Verification items for the finished model (mm, model axes). Face numbers are marked on the shaded views. Round coordinates to 2 decimals unless told otherwise and drop trailing zeros. Order: outer loops, then holes, each group sorted by start corner. A loop starts at its lowest first (then second) coordinate and runs counter-clockwise, first axis right, second up. Notation, with made-up numbers: M 62,6.25 L 66,6.25 A24 cw 66,44.25 Z; hole C 72.25,-4 d8. An arc over 180 degrees is marked long. Answer as a JSON object with one key per item and string values. Group by question number.
```python
from build123d import *

# Parameters (mm, degrees)
F1_DEPTH  = 7.1
F2_T      = -2.5
F4_DEPTH  = 25
F5_W      = 12.5
F5_H      = 1.25
F6_DEPTH  = 2.5
F7_W      = 23.5
F7_H      = 1.25
F8_DEPTH  = 2.5
F9_W      = 1.5
F9_H      = 7.25
F9_R      = 2.5
F10_DEPTH = 4.4


with BuildPart() as f1:
    # F0 (on Front) → F1 (new body)
    with BuildSketch(Plane.XZ):
        with BuildLine():
            Line((68.55, 39.5), (-68.55, 39.5))
            ThreePointArc((-68.55, 39.5), (-72.72193, 37.77193), (-74.45, 33.6))
            Line((-74.45, 33.6), (-74.45, -33.6))
            ThreePointArc((-74.45, -33.6), (-72.72193, -37.77193), (-68.55, -39.5))
            Line((-68.55, -39.5), (68.55, -39.5))
            ThreePointArc((68.55, -39.5), (72.72193, -37.77193), (74.45, -33.6))
            Line((74.45, -33.6), (74.45, 33.6))
            ThreePointArc((74.45, 33.6), (72.72193, 37.77193), (68.55, 39.5))
        make_face()
    extrude(amount=-F1_DEPTH)

    # F2
    f2_openings = [f1.faces().sort_by_distance(p)[0] for p in [
        (0, 0, 0),
    ]]
    offset(amount=F2_T, openings=f2_openings)

    # F3 (on Front) → F4 (cut)
    with BuildSketch(Plane.XZ):
        Polygon((60.65, 21.3), (44.45, 21.3), (44.45, 0), (44.45, -21.3), (60.65, -21.3), (60.65, 0), align=None)
    extrude(amount=-F4_DEPTH, mode=Mode.SUBTRACT)

    # F5 (on face) → F6 (cut)
    with BuildSketch(Plane(origin=(0, 0, -39.5), x_dir=(1, 0, 0), z_dir=(0, 0, -1))):
        with Locations((30.7, -3.245512)):
            Rectangle(F5_W, F5_H)
        with Locations((30.7, -4.495512)):
            Rectangle(F5_W, F5_H)
    extrude(amount=-F6_DEPTH, mode=Mode.SUBTRACT)

    # F7 (on face) → F8 (cut)
    with BuildSketch(Plane.XY.offset(39.5)):
        with Locations((38.7, 2.925)):
            Rectangle(F7_W, F7_H)
        with Locations((38.7, 4.175)):
            Rectangle(F7_W, F7_H)
    extrude(amount=-F8_DEPTH, mode=Mode.SUBTRACT)

    # F9 (on face) → F10 (cut)
    with BuildSketch(Plane(origin=(-74.45, 0, 0), x_dir=(0, -1, 0), z_dir=(-1, 0, 0))):
        with Locations((-4.3, -3.625)):
            Rectangle(F9_W, F9_H)
        with Locations((-2.8, -3.625)):
            Rectangle(F9_W, F9_H)
        Polygon((-3.55, 0), (-2.05, 0), (-2.05, 7.25), (-3.55, 7.25), (-5.05, 7.25), (-5.05, 0), align=None)
        with Locations((-3.55, 20.8)):
            Circle(F9_R)
    extrude(amount=-F10_DEPTH, mode=Mode.SUBTRACT)


solid = f1.part
```
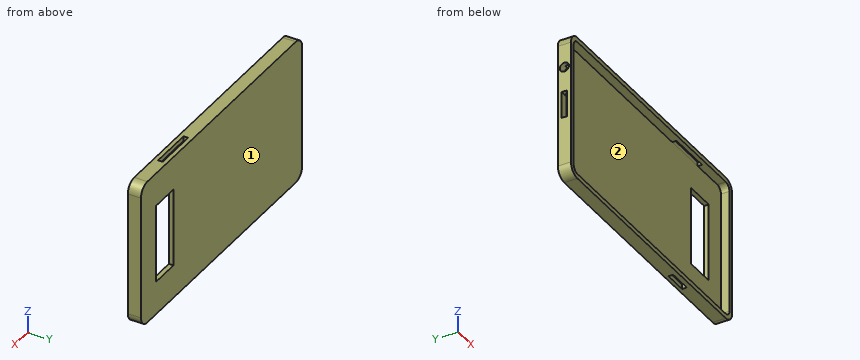
Q1. Cross-section at A-A, the plane z = 4.5. Record the cut outline in (x, y), then the cut area to 3 significant figures.
Q2. Cross-section at B-B, the plane z = -10. Record the cut outline in (x, y).
Q3. Thickness scan on line 1 (Z direction, x = 12, y = 3.75); line 2 (X direction, y = 1.25, z = 8); line 3 (X direction, y = 6.25, z = -13). Record the ranges inside material, lowest first. Write a range as from..to.
Q4. Release check for a two-part mould opening along Z. For the marked faces 1 and 2 record: released by +Z, released by -Z, zero draft, split by the parting line, or undercut.
Q5. Gauge pin test, flat ends, axial feed: pin 1 Ø4 at (x, z) = (4.5, -20) entering from -Y; pin 2 Ø2 at (x, z) = (34, -38) entering from -Y; pin 3 Ø4 at (y, z) = (3.55, 20.8) entering from -X; pin 4 Ø3 at (y, z) = (3.5, 37.5) entering from -X. Record the tip position at first contact, or that the pin passes through.
Q6. Cross-section at C-C, the plane x = -6.5. Record the cut outline in (y, z), then the cut area to 4 significant figures.
Q7. Cross-section at D-D, the plane z = -32. Record the cut outline in (x, y), then the cut area to 3 significant figures.
Conclusion:
{
 "1": {"outline": "M -74.45,0 L -71.95,0 L -71.95,2.05 L -74.45,2.05 Z; M -74.45,5.05 L -70.05,5.05 L -70.05,4.6 L 44.45,4.6 L 44.45,7.1 L -74.45,7.1 Z; M 60.65,4.6 L 71.95,4.6 L 71.95,0 L 74.45,0 L 74.45,7.1 L 60.65,7.1 Z", "area": "346 mm2"},
 "2": {"outline": "M -74.45,0 L -71.95,0 L -71.95,4.6 L 44.45,4.6 L 44.45,7.1 L -74.45,7.1 Z; M 60.65,4.6 L 71.95,4.6 L 71.95,0 L 74.45,0 L 74.45,7.1 L 60.65,7.1 Z"},
 "3": {"line 1": "-39.5..-37, 37..39.5", "line 2": "-74.45..-71.95, 71.95..74.45", "line 3": "-74.45..44.45, 60.65..74.45"},
 "4": {"face 1": "zero draft", "face 2": "undercut"},
 "5": {"pin 1": "y = 4.6", "pin 2": "y = 0", "pin 3": "x = -70.05", "pin 4": "x = -73.94"},
 "6": {"outline": "M 0,-39.5 L 7.1,-39.5 L 7.1,39.5 L 0,39.5 L 0,37 L 4.6,37 L 4.6,-37 L 0,-37 Z", "area": "220.5 mm2"},
 "7": {"outline": "M -74.45,0 L -71.95,0 L -71.95,4.6 L 71.95,4.6 L 71.95,0 L 74.45,0 L 74.45,7.1 L -74.45,7.1 Z", "area": "395 mm2"}
}
